Design review of the part built by this model. Coordinates are the model's own, in mm. A direction names the side the tool comes from. Coordinates: 2 decimals unless noted, no trailing zeros. Loops run counter-clockwise (first coordinate to the right, second up) from the corner with the lowest first, then second, coordinate; pieces in that order, holes last.
Q1. Machinability: for faces 4 (the face through (-1, 23, 35.263)), 5 (the face through (-50.226, 23, 0)), 6 (the face through (50.226, 23, 0)), which of the approach directions +Z, -Z, +X, -X, +Y, -Y give a long, thin tool a straight path to every point of the face, cutting with its end or side? Answer none if there is none.
Q2. For P1, Ø8, axis at x = 55, z = 39.52, coming from the +Y side; P2, Ø8, axis at x = -1, y = 22.5, coming from the -Z side; P3, Ø3, axis at y = 21.5, z = 28, coming from the +X side; P4, Ø1.5, axis at y = 19, z = 21, coming from the -X side, all flat-tipped, find the tip position at first contact; note any pin that passes through.
Q3. Wall thickness on probe 1 along Z at (x, y) = (-53, 7.5); probe 2 along X at (y, z) = (12.5, 41); probe 3 along X at (y, z) = (9.25, -38): over which ranges is each line inside the solid? List them lowest first.
Q4. Add section B-B on x = -31. Give the boundary of the cut face in (y, z).
Q5. Add section A-A on z = 41.5. Give the boundary of the cut face in (x, y), and give its area (3 significant figures).
Q6. Add section D-D on z = -7.5. Give the boundary of the cut face in (x, y), and give its area (3 significant figures).
Q7. Add section C-C on y = 21. Give the boundary of the cut face in (x, z).
Q8. Draft analysis for pull direction Z (two halves, no side actions). For faces 1 (the face through (-1, 9, -55)), 2 (the face through (-1, 28, 0)), 3 (the face through (-51.38, 8.87, 36.78)), state which applies: released by +Z, released by -Z, zero draft, split by the parting line, or undercut.
```python
from build123d import *

# Parameters (mm, degrees)
F_01_BASE_PROFILE_W           = 150
F_01_BASE_PROFILE_H           = 110
F_01_BASE_PROFILE_R           = 3.711604984
F_01_BASE_PROFILE_R_2         = 4.5
F_01_BASE_PROFILE_R_3         = 1.223591395
F_01_BASE_PROFILE_R_4         = 5.612716763
F_01_BASE_PROFILE_W_2         = 70
F_01_BASE_PROFILE_H_2         = 24
F_01_BASE_EXTRUDE_DEPTH       = 18
F_02_BOSS_PROFILE_W           = 100.452577252
F_02_BOSS_PROFILE_H           = 70.52593178
F_02_REINFORCEMENT_BOSS_DEPTH = 28


with BuildPart() as part:
    # 01_Base_Profile → 01_Base_Extrude (new body)
    with BuildSketch(Plane(origin=(0, 0, 0), x_dir=(1, 0, 0), z_dir=(0, 1, 0))):
        Rectangle(F_01_BASE_PROFILE_W, F_01_BASE_PROFILE_H)
        with Locations(Location((-53.887283237, -39.51734104, 0), (0, 0, 270))):
            Circle(F_01_BASE_PROFILE_R, mode=Mode.SUBTRACT)
        with Locations(Location((55, -39.51734104, 0), (0, 0, 270))):
            Circle(F_01_BASE_PROFILE_R_2, mode=Mode.SUBTRACT)
        with Locations(Location((-53.887283237, 38, 0), (0, 0, 270))):
            Circle(F_01_BASE_PROFILE_R_3, mode=Mode.SUBTRACT)
        with Locations(Location((53.887283237, 39.51734104, 0), (0, 0, 270))):
            Circle(F_01_BASE_PROFILE_R_4, mode=Mode.SUBTRACT)
        Rectangle(F_01_BASE_PROFILE_W_2, F_01_BASE_PROFILE_H_2, mode=Mode.SUBTRACT)
    extrude(amount=F_01_BASE_EXTRUDE_DEPTH)

    # 02_Boss_Profile → 02_Reinforcement_Boss (add)
    with BuildSketch(Plane(origin=(0, 0, 0), x_dir=(1, 0, 0), z_dir=(0, 1, 0))):
        Rectangle(F_02_BOSS_PROFILE_W, F_02_BOSS_PROFILE_H)
    extrude(amount=F_02_REINFORCEMENT_BOSS_DEPTH)


solid = part.part
```
Entries:
1. face 4: +Z, +X, -X, +Y
1. face 5: +Z, -Z, -X, +Y
1. face 6: +Z, -Z, +X, +Y
2. P1: passes through
2. P2: stops at z = -35.26
2. P3: stops at x = 50.23
2. P4: stops at x = -50.23
3. probe 1: z = -55 to -38.84, -37.16 to 35.91, 43.12 to 55
3. probe 2: x = -75 to -57.29, -50.48 to 50.75, 59.25 to 75
3. probe 3: x = -75 to -55.11, -52.66 to 48.48, 59.29 to 75
4. outline: (0, -55) - (18, -55) - (18, -35.26) - (28, -35.26) - (28, 35.26) - (18, 35.26) - (18, 55) - (0, 55) - close
5. outline: (-75, 0) - (-57.02, 0) - (-57.02, 18) - (-75, 18) - close; (-50.75, 0) - (50.96, 0) - (50.96, 18) - (-50.75, 18) - close; (59.04, 0) - (75, 0) - (75, 18) - (59.04, 18) - close
5. area: 2,440 mm2
6. outline: (-75, 0) - (75, 0) - (75, 18) - (50.23, 18) - (50.23, 28) - (-50.23, 28) - (-50.23, 18) - (-75, 18) - close
6. area: 3,700 mm2
7. outline: (-50.23, -35.26) - (50.23, -35.26) - (50.23, 35.26) - (-50.23, 35.26) - close
8. face 1: released by -Z
8. face 2: zero draft
8. face 3: undercut
